```python
from build123d import *

# Parameters (mm, degrees)
F0_R     = 9.525
F1_DEPTH = 19.05
F2_R     = 3.175
F3_DEPTH = 3.175
F4_R     = 3.175
F5_DEPTH = 3.175
F6_SIZE  = 0.254
F7_R     = 2.38125
F8_DEPTH = 12.7


with BuildPart() as f1:
    # F0 (on Top) → F1 (new body)
    with BuildSketch(Plane.XY):
        Circle(F0_R)
    extrude(amount=F1_DEPTH)

    # F2 (on face) → F3 (join)
    with BuildSketch(Plane(origin=(0, 0, 0), x_dir=(1, 0, 0), z_dir=(0, 0, -1))):
        Circle(F2_R)
    extrude(amount=F3_DEPTH)

    # F4 (on face) → F5 (join)
    with BuildSketch(Plane.XY.offset(19.05)):
        Circle(F4_R)
    extrude(amount=F5_DEPTH)

    # F6
    f6_edges = [f1.edges().sort_by_distance(p)[0] for p in [
        (-9.525, 0, 19.05),
        (-3.175, 0, -3.175),
        (-9.525, 0, 0),
        (-3.175, 0, 22.225),
    ]]
    chamfer(f6_edges, length=F6_SIZE)

    # F7 (on Right) → F8 (cut, symmetric)
    with BuildSketch(Plane.YZ):
        with Locations((0, 9.525)):
            Circle(F7_R)
    extrude(amount=F8_DEPTH, both=True, mode=Mode.SUBTRACT)


solid = f1.part
```
Model file for the job. Use its own axes, mm. A direction names the side the tool comes from. Round coordinates to 2 decimals unless told otherwise and drop trailing zeros. Loops run counter-clockwise (first coordinate to the right, second up) from the corner with the lowest first, then second, coordinate; pieces in that order, holes last. Notation, with made-up numbers: M 32.25,-9.75 L 80.25,-9.75 A15 ccw 80.25,2.25 Z; hole C 33.5,32 d3. An arc over 180 degrees is marked long. Put each result on its own line as item: value. Start each with the question number.
Item 1: Mould opens along Y. For faces 1 (the face through (0.133, -0.31, 11.886)), 2 (the face through (9.085, 2.861, 9.395)), 3 (the face through (0, 0, 22.225)) say: released by +Y, released by -Y, zero draft, split by the parting line, or undercut.
Item 2: Cut at C-C (z = 4.5). List the corners of the cut face in (x, y) (3 decimals), then the cut area to 3 significant figures.
Item 3: Drop flat-ended pins along their axis: P1, Ø4, axis at x = -6, z = 17.5, coming from the -Y side; P2, Ø5, axis at x = 3.5, y = 6, coming from the -Z side; P3, Ø10, axis at x = -7.5, z = 15.5, coming from the +Y side. Give the stop position or say it passes through.
Item 4: Drill centre lines: line 1 along Z through (x, y) = (3.75, 0); line 2 along Z through (x, y) = (-2.25, 0) (3 decimals); line 3 along Z through (x, y) = (-0.5, -3.25). Where is each one in solid material? Low to high.
Item 5: Cut at B-B (y = 0). List the corners of the cut face in (x, z) (3 decimals), then the cut area to 3 significant figures.
Item 6: 3-axis set-ups, long thin cutter, end or side, ignore diameter. For faces 4 (the face through (-0.69, 3.1, -1.44)), 5 (the face through (0, 0, -3.175)), 6 (the face through (-0.69, -3.1, 20.49)): which of +Z, -Z, +X, -X, +Y, -Y reach the whole face in a straight line?
Answer block:
1. face 1: undercut
1. face 2: split by the parting line
1. face 3: zero draft
2. outline: C 0,0 d19.05
2. area: 285 mm2
3. P1: y = -8.64
3. P2: z = 0
3. P3: y = 9.19
4. line 1: 0 to 7.14, 11.91 to 19.05
4. line 2: -3.175 to 7.144, 11.906 to 22.225
4. line 3: 0 to 19.05
5. outline: M -9.525,0.254 L -9.271,0 L -3.175,0 L -3.175,-2.921 L -2.921,-3.175 L 2.921,-3.175 L 3.175,-2.921 L 3.175,0 L 9.271,0 L 9.525,0.254 L 9.525,7.144 L -9.525,7.144 Z; M -9.525,11.906 L 9.525,11.906 L 9.525,18.796 L 9.271,19.05 L 3.175,19.05 L 3.175,21.971 L 2.921,22.225 L -2.921,22.225 L -3.175,21.971 L -3.175,19.05 L -9.271,19.05 L -9.525,18.796 Z
5. area: 312 mm2
6. face 4: -Z
6. face 5: -Z, +X, -X, +Y, -Y
6. face 6: +Z
